Part model, mm, in its own coordinate system. Face numbers are marked on the shaded views. A direction names the side the tool comes from. Coordinates: 2 decimals unless noted, no trailing zeros. Loops run counter-clockwise (first coordinate to the right, second up) from the corner with the lowest first, then second, coordinate; pieces in that order, holes last. Notation, with made-up numbers: (-27.75, 8) - (-10.75, 8) arc R15 ccw to (-10.75, 14) - close; hole circle Ø5 at (37.25, 38). An arc over 180 degrees is marked (long way). Use a Markdown table: item, result. Add a question column.
1) Pull direction Z, two halves, no side cores. Call the marked faces 1, 2 and 3: +Z half, -Z half, draft (parallel to the pull), parting line (faces both ways), or undercut.
2) Probe probe 1 along Y at (x, z) = (1.75, -1.25); probe 2 along X at (y, z) = (15.5, -0.25); probe 3 along Z at (x, y) = (-1.75, 6.25). List the from-to ranges inside material, lowest first. Write a range as [from, to].
3) Band-saw the part on B-B (y = 9.5). Give the cut face in (x, z).
4) Tool access for the marked faces 4, 5 and 6: list every direction of +Z, -Z, +X, -X, +Y, -Y with a clear straight run to the whole face (end or side of a thin tool).
5) Drop flat-ended pins along their axis: P1, Ø0.8, axis at x = -1, y = 16, coming from the +Z side; P2, Ø2, axis at x = -2, y = 5.5, coming from the +Z side; P3, Ø1, axis at x = -2, y = 2.5, coming from the +Z side. Give the stop position or say it passes through.
from build123d import *

# Parameters (mm, degrees)
SKETCH_1_R          = 2
EXTRUDE_1_DEPTH     = 14
SKETCH_2_R          = 3.3
EXTRUDE_2_DEPTH     = 2.7
FILLET_1_R          = 1
CHAMFER_1_SIZE      = 0.5
SKETCH_3_W          = 4
SKETCH_3_H          = 1
SKETCH_3_W_2        = 1
SKETCH_3_H_2        = 4
CUT_EXTRUDE_1_DEPTH = 1
CHAMFER_2_SIZE      = 1


with BuildPart() as part:
    # 草图1 → 凸台-拉伸1 (new body)
    with BuildSketch(Plane(origin=(0, 0, 0), x_dir=(1, 0, 0), z_dir=(0, 1, 0))):
        with Locations(Location((0, 0, 0), (0, 0, 270))):
            Circle(SKETCH_1_R)
    extrude(amount=EXTRUDE_1_DEPTH)

    # 草图2 → 凸台-拉伸2 (add)
    with BuildSketch(Plane(origin=(0, 14, 0), x_dir=(1, 0, 0), z_dir=(0, 1, 0))):
        with Locations(Location((0, 0, 0), (0, 0, 90))):
            Circle(SKETCH_2_R)
    extrude(amount=EXTRUDE_2_DEPTH)

    # 圆角1
    fillet_1_edges = [part.edges().sort_by_distance(p)[0] for p in [
        (0, 16.7, 3.3),
    ]]
    fillet(fillet_1_edges, radius=FILLET_1_R)

    # 倒角1
    chamfer_1_edges = [part.edges().sort_by_distance(p)[0] for p in [
        (0, 0, -2),
    ]]
    chamfer(chamfer_1_edges, length=CHAMFER_1_SIZE)

    # 草图3 → 切除-拉伸-薄壁1 (cut)
    with BuildSketch(Plane(origin=(0, 16.7, 0), x_dir=(1, 0, 0), z_dir=(0, 1, 0))):
        Rectangle(SKETCH_3_W, SKETCH_3_H)
        Rectangle(SKETCH_3_W_2, SKETCH_3_H_2)
    extrude(amount=-CUT_EXTRUDE_1_DEPTH, mode=Mode.SUBTRACT)

    # 倒角2
    chamfer_2_edges = [part.edges().sort_by_distance(p)[0] for p in [
        (0, 15.7, 2),
        (2, 15.7, 0),
        (0, 15.7, -2),
        (-2, 15.7, 0),
    ]]
    chamfer(chamfer_2_edges, length=CHAMFER_2_SIZE - 0.0001)  # a hair under: the kernel refuses the full size


solid = part.part
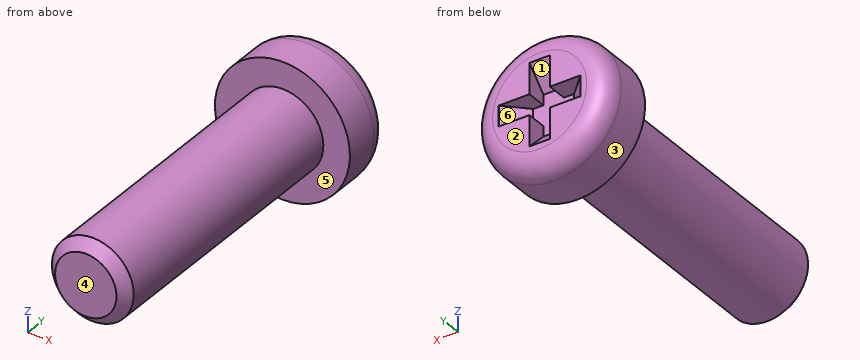
Answer block:
| question | item | result |
|---|---|---|
| 1 | face 1 | undercut |
| 1 | face 2 | draft |
| 1 | face 3 | parting line |
| 2 | probe 1 | [14, 16.7] |
| 2 | probe 2 | [-3.29, 3.29] |
| 2 | probe 3 | [-0.97, 0.97] |
| 3 | outline | circle Ø4 at (0, 0) |
| 4 | face 4 | +Z, -Z, +X, -X, -Y |
| 4 | face 5 | -Y |
| 4 | face 6 | +Y |
| 5 | P1 | z = 3.23 |
| 5 | P2 | z = 1.73 |
| 5 | P3 | z = 1.32 |
